Geometry check sheet. Reference: the model listing, model coordinates, mm. Face numbers are marked on the shaded views. A direction names the side the tool comes from. Coordinates: 2 decimals unless noted, no trailing zeros. Write each loop counter-clockwise with the first axis right and the second up, starting at its lowest first coordinate (ties: lowest second). Pieces come first, ordered by that corner, then holes. Notation, with made-up numbers: (11, -12) -> (29, -12) arc R29 cw to (29, 26) -> close; hole circle Ø10 at (75.5, -3.5). An arc over 180 degrees is marked (long way). Use a Markdown table: item, result.
```python
from build123d import *

# Parameters (mm, degrees)
PAD_DEPTH     = 10
SKETCH001_R   = 6
SKETCH001_R_2 = 3.8
PAD001_DEPTH  = 2


with BuildPart() as part:
    # Sketch → Pad (new body)
    with BuildSketch(Plane.XY):
        with BuildLine():
            Line((-55.40988, 26.565392), (-30.40988, 26.565392))
            ThreePointArc((-30.40988, 12.565392), (-15.753026, 19.565392), (-30.40988, 26.565392))
            Line((-30.40988, 12.565392), (-55.40988, 12.565392))
            Line((-55.40988, 12.565392), (-55.40988, 15.515392))
            Line((-55.40988, 15.515392), (-33.40988, 15.515392))
            Line((-33.40988, 15.515392), (-33.40988, 23.615392))
            Line((-55.40988, 23.615392), (-33.40988, 23.615392))
            Line((-55.40988, 26.565392), (-55.40988, 23.615392))
        make_face()
        Polygon((-20.422899, 22.065392), (-20.422899, 17.065392), (-24.753026, 14.565392), (-29.083153, 17.065392), (-29.083153, 22.065392), (-24.753026, 24.565392), align=None, mode=Mode.SUBTRACT)
    extrude(amount=PAD_DEPTH)

    # Sketch001 → Pad001 (new body)
    with BuildSketch(Plane(origin=(0, 0, 0), x_dir=(1, 0, 0), z_dir=(0, 0, -1))):
        with Locations((-24.70988, -19.565392)):
            Circle(SKETCH001_R)
        with Locations((-24.70988, -19.565392)):
            Circle(SKETCH001_R_2, mode=Mode.SUBTRACT)
    extrude(amount=-PAD001_DEPTH)


solid = part.part
```
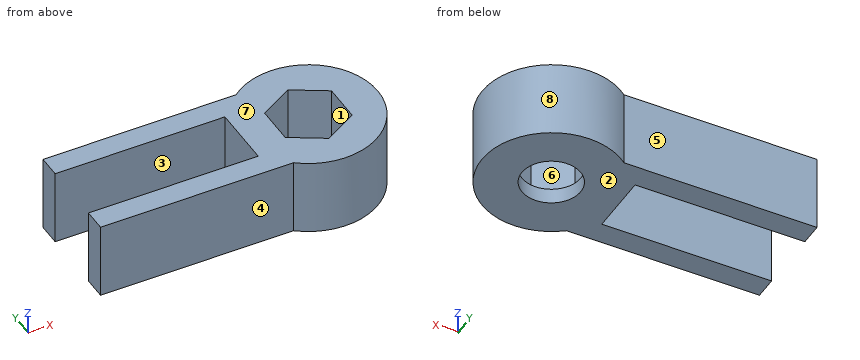
Item 1: Section check D-D on x = -31. Record the boundary of the cut face in (y, z), then the cut area to 3 significant figures.
Answer block:
| item | result |
|---|---|
| outline | (12.57, 0) -> (26.57, 0) -> (26.57, 10) -> (12.57, 10) -> close |
| area | 140 mm^2 |
Item 2: Tool access check on the marked faces 1, 2, 3 and 4. Record the directions out of +Z, -Z, +X, -X, +Y, -Y that give a thin tool (end or side, any length) a straight path to the whole face; none if there is none.
Answer block:
| item | result |
|---|---|
| face 1 | +Z |
| face 2 | -Z, +X, -X, +Y, -Y |
| face 3 | +Z, -Z, -X |
| face 4 | +Z, -Z, -X, -Y |
Item 3: Section check C-C on y = 17.75. Record the boundary of the cut face in (x, z).
Answer block:
| item | result |
|---|---|
| outline | (-33.41, 0) -> (-28.05, 0) -> (-28.05, 2) -> (-29.08, 2) -> (-29.08, 10) -> (-33.41, 10) -> close; (-21.37, 0) -> (-15.94, 0) -> (-15.94, 10) -> (-20.42, 10) -> (-20.42, 2) -> (-21.37, 2) -> close |
Item 4: Depth check by flat-ended pin: P1, Ø4, axis at y = 23.5, z = 7.5, coming from the -X side; P2, Ø5, axis at x = -44.5, z = 7, coming from the +Y side; P3, Ø2, axis at x = -21, z = 6, coming from the +Y side; P4, Ø2.5, axis at y = 19.5, z = 6.5, coming from the -X side. Enter the tip coordinate at first touch or a pass-through.
Answer block:
| item | result |
|---|---|
| P1 | stops at x = -55.41 |
| P2 | stops at y = 26.57 |
| P3 | stops at y = 28.13 |
| P4 | stops at x = -33.41 |
Item 5: Section check B-B on z = 8.75. Record the boundary of the cut face in (x, y).
Answer block:
| item | result |
|---|---|
| outline | (-55.41, 12.57) -> (-30.41, 12.57) arc R9 ccw (long way) to (-30.41, 26.57) -> (-55.41, 26.57) -> (-55.41, 23.62) -> (-33.41, 23.62) -> (-33.41, 15.52) -> (-55.41, 15.52) -> close; hole (-29.08, 17.07) -> (-24.75, 14.57) -> (-20.42, 17.07) -> (-20.42, 22.07) -> (-24.75, 24.57) -> (-29.08, 22.07) -> close |
Item 6: Section check A-A on x = -37. Record the boundary of the cut face in (y, z), then the cut area to 3 significant figures.
Answer block:
| item | result |
|---|---|
| outline | (12.57, 0) -> (15.52, 0) -> (15.52, 10) -> (12.57, 10) -> close; (23.62, 0) -> (26.57, 0) -> (26.57, 10) -> (23.62, 10) -> close |
| area | 59.0 mm^2 |
Item 7: Mould release check, pull along Y, two halves, no side actions. Record for the marked faces 5, 6, 7 and 8: +Y half, -Y half, draft (parallel to the pull), parting line (faces both ways), or undercut.
Answer block:
| item | result |
|---|---|
| face 5 | +Y half |
| face 6 | undercut |
| face 7 | draft |
| face 8 | parting line |
Item 8: Thickness scan on L1, parallel to Y at x = -47.5, z = 1; L2, parallel to Z at x = -28, y = 22; L3, parallel to X at y = 16.25, z = 8.75. Record the ranges inside material, lowest first. Write a range as [from, to].
Answer block:
| item | result |
|---|---|
| L1 | y = [12.57, 15.52], [23.62, 26.57] |
| L2 | z = [0, 2] |
| L3 | x = [-33.41, -27.67], [-21.84, -16.39] |
